Part model, mm, in its own coordinate system. A direction names the side the tool comes from. Give positions to 0.01 mm unless a question says otherwise; leave off trailing zeros. Write each loop counter-clockwise with the first axis right and the second up, starting at its lowest first coordinate (ties: lowest second). Pieces come first, ordered by that corner, then holes.
```python
from build123d import *

# Parameters (mm, degrees)
SKETCH1_R           = 2.125
BOSS_EXTRUDE1_DEPTH = 1
BOSS_EXTRUDE1_TAPER = 3
SKETCH2_R           = 2.95
BOSS_EXTRUDE2_DEPTH = 0.5
SKETCH3_R           = 0.25
CUT_EXTRUDE1_DEPTH  = 5.43339599


with BuildPart() as part:
    # Sketch1 → Boss-Extrude1 (new body)
    with BuildSketch(Plane(origin=(0, 0, 0), x_dir=(1, 0, 0), z_dir=(0, 1, 0))):
        Circle(SKETCH1_R)
    extrude(amount=BOSS_EXTRUDE1_DEPTH, taper=BOSS_EXTRUDE1_TAPER)

    # Sketch2 → Boss-Extrude2 (add)
    with BuildSketch(Plane.XZ):
        with Locations(Location((0, 0, 0), (0, 0, 270))):
            Circle(SKETCH2_R)
    extrude(amount=BOSS_EXTRUDE2_DEPTH)

    # Sketch3 → Cut-Extrude1 (cut, through all)
    with BuildSketch(Plane(origin=(0, 1, 0), x_dir=(1, 0, 0), z_dir=(0, 1, 0))):
        with Locations(Location((0, 0, 0), (0, 0, 270))):
            Circle(SKETCH3_R)
    extrude(amount=-CUT_EXTRUDE1_DEPTH, mode=Mode.SUBTRACT)


solid = part.part
```
1) Saw through at D-D, the plane x = 2.5. Write the cut outline in (y, z).
Answers follow:
outline: (-0.5, -1.57) - (0, -1.57) - (0, 1.57) - (-0.5, 1.57) - close
2) 3-axis set-ups, long thin cutter, end or side, ignore diameter. For faces 1 (the face through (-1.9, 0, -1.3)), 2 (the face through (-2.88, -0.25, 0.64)): which of +Z, -Z, +X, -X, +Y, -Y reach the whole face in a straight line?
Answers follow:
face 1: +Y
face 2: +Y, -Y
3) Saw through at B-B, the plane y = -0.4. Write the cut outline in (x, z), then the cut area to 3 significant figures.
Answers follow:
outline: circle Ø5.9 at (0, 0); hole circle Ø0.5 at (0, 0)
area: 27.1 mm2
4) Saw through at C-C, the plane z = -2.5. Write the cut outline in (x, y).
Answers follow:
outline: (-1.57, -0.5) - (1.57, -0.5) - (1.57, 0) - (-1.57, 0) - close
5) Wall check: L1, parallel to Y at x = 0.1, z = 2.4; L2, parallel to X at y = 0.1, z = -0.1; L3, parallel to X at y = -0.2, z = -0.15. Give the ranges that are in metal, low to high.
Answers follow:
L1: y = -0.5 to 0
L2: x = -2.12 to -0.23, 0.23 to 2.12
L3: x = -2.95 to -0.2, 0.2 to 2.95
6) Saw through at A-A, the plane x = 0. Write the cut outline in (y, z) (3 decimals).
Answers follow:
outline: (-0.5, -2.95) - (0, -2.95) - (0, -2.125) - (1, -2.073) - (1, -0.25) - (-0.5, -0.25) - close; (-0.5, 0.25) - (1, 0.25) - (1, 2.073) - (0, 2.125) - (0, 2.95) - (-0.5, 2.95) - close
